Build history of the part. All positions in model axes, mm. Give positions to 0.01 mm unless a question says otherwise; leave off trailing zeros. Write each loop counter-clockwise with the first axis right and the second up, starting at its lowest first coordinate (ties: lowest second). Pieces come first, ordered by that corner, then holes. Notation, with made-up numbers: (70, -31) -> (87, -31) arc R11 cw to (87, -12) -> close; hole circle Ø1 at (88.5, 54). An arc over 180 degrees is marked (long way). Write item = value, one per line. Start each with the question number.
Q1. Wall check: line 1 (X direction, y = 1529.5, z = 4610.5); line 2 (Z direction, x = -2205.5, y = 1530); line 3 (Z direction, x = -2558, y = 1538). Give the ranges that are in metal, low to high.
Q2. Saw through at A-A, the plane x = -2200. List the corners of the cut face in (y, z).
Q3. Saw through at B-B, the plane z = 4727.5. List the corners of the cut face in (x, y), then the cut area to 3 significant figures.
Q4. Saw through at D-D, the plane x = -2770. List the corners of the cut face in (y, z).
Q5. Saw through at C-C, the plane y = 1539. List the corners of the cut face in (x, z).
Q6. Drop flat-ended pins along their axis: P1, Ø5, axis at x = -2745, y = 1558, coming from the -Z side; P2, Ø15, axis at x = -2521, y = 1544.5, coming from the -Z side; P3, Ø2, axis at x = -2363, y = 1547.5, coming from the +Z side. Give the stop position or say it passes through.
from build123d import *

# Parameters (mm, degrees)
PAD018_DEPTH    = 50
POCKET003_DEPTH = 59
SKETCH022_W     = 780.912842
SKETCH022_H     = 501.60791
POCKET004_DEPTH = 60
SKETCH021_W     = 824.843506
SKETCH021_H     = 493.205078
POCKET005_DEPTH = 60


with BuildPart() as part:
    # Sketch023 → Pad018 (new body)
    with BuildSketch(Plane.XZ):
        Polygon((-3036.804688, 4960.135254), (-3036.804688, 3429.500488), (-2339.515625, 2587.651367), (-2050.395752, 2587.651367), (-2050.395752, 4960.135254), align=None)
    extrude(amount=PAD018_DEPTH)

    # Sketch024 (on Face7 of Pad018) → Pocket003 (cut)
    with BuildSketch(Plane.XZ.offset(50)):
        Polygon((-2794.763916, 3478.686768), (-2263.660645, 2821.494141), (-2263.660645, 3478.686768), align=None)
    extrude(amount=-POCKET003_DEPTH, mode=Mode.SUBTRACT)

    # Sketch022 (on Face5 of Pocket003) → Pocket004 (cut)
    with BuildSketch(Plane.XZ.offset(50)):
        with Locations((-2555.920776, 4033.548584)):
            Rectangle(SKETCH022_W, SKETCH022_H)
    extrude(amount=-POCKET004_DEPTH, mode=Mode.SUBTRACT)

    # Sketch021 (on Face5 of Pocket004) → Pocket005 (cut)
    with BuildSketch(Plane.XZ.offset(50)):
        with Locations((-2560.651733, 4738.429199)):
            Rectangle(SKETCH021_W, SKETCH021_H)
    extrude(amount=-POCKET005_DEPTH, mode=Mode.SUBTRACT)


with BuildPart() as part_1:
    # Body016 placement: moved
    add(part.part.moved(Location((0, 1572, 0))))


solid = part_1.part
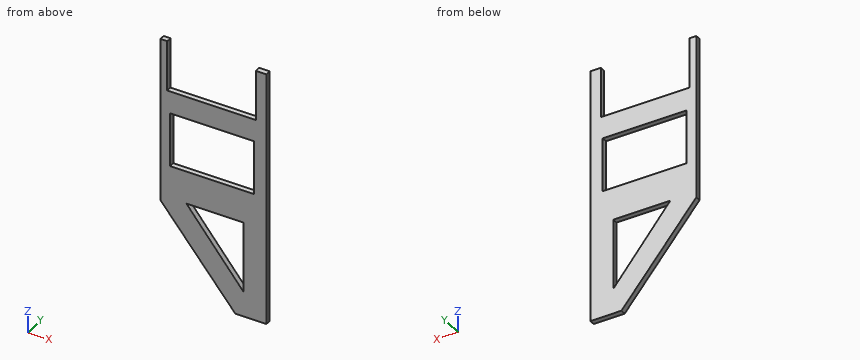
Report:
q1.line_1 = -3036.8 to -2973.07, -2148.23 to -2050.4
q1.line_2 = 2587.65 to 3782.74, 4284.35 to 4491.83
q1.line_3 = 2851.43 to 3185.71, 3478.69 to 3782.74, 4284.35 to 4491.83
q2.outline = (1522, 2587.65) -> (1572, 2587.65) -> (1572, 3782.74) -> (1522, 3782.74) -> close; (1522, 4284.35) -> (1572, 4284.35) -> (1572, 4491.83) -> (1522, 4491.83) -> close
q3.outline = (-3036.8, 1522) -> (-2973.07, 1522) -> (-2973.07, 1572) -> (-3036.8, 1572) -> close; (-2148.23, 1522) -> (-2050.4, 1522) -> (-2050.4, 1572) -> (-2148.23, 1572) -> close
q3.area = 8,080 mm2
q4.outline = (1522, 3107.38) -> (1572, 3107.38) -> (1572, 3448.04) -> (1522, 3448.04) -> close; (1522, 3478.69) -> (1572, 3478.69) -> (1572, 3782.74) -> (1522, 3782.74) -> close; (1522, 4284.35) -> (1572, 4284.35) -> (1572, 4491.83) -> (1522, 4491.83) -> close
q5.outline = (-3036.8, 3429.5) -> (-2339.52, 2587.65) -> (-2050.4, 2587.65) -> (-2050.4, 4960.14) -> (-2148.23, 4960.14) -> (-2148.23, 4491.83) -> (-2973.07, 4491.83) -> (-2973.07, 4960.14) -> (-3036.8, 4960.14) -> close; hole (-2946.38, 3782.74) -> (-2165.46, 3782.74) -> (-2165.46, 4284.35) -> (-2946.38, 4284.35) -> close; hole (-2794.76, 3478.69) -> (-2263.66, 2821.49) -> (-2263.66, 3478.69) -> close
q6.P1 = 3074.18
q6.P2 = 2797.71
q6.P3 = 4491.83
